from build123d import *

# Parameters (mm, degrees)
ESQUISSE1_R             = 10
BOSS_EXTRU_1_DEPTH      = 1
ESQUISSE2_R             = 6.25
BOSS_EXTRU_2_DEPTH      = 2.5
ESQUISSE3_R             = 3.25
ENL_V_MAT_EXTRU_1_DEPTH = 15.568802284
CHANFREIN1_SIZE         = 0.2


with BuildPart() as part:
    # Esquisse1 → Boss.-Extru.1 (new body)
    with BuildSketch(Plane(origin=(38.31198223, 224.2058109, 0), x_dir=(0.9566700248572155, 0.2911742837884119, 0), z_dir=(0, 0, -1))):
        with Locations(Location((-101.934891402, 203.3355147, 0), (0, 0, 196.92827176))):
            Circle(ESQUISSE1_R)
    extrude(amount=BOSS_EXTRU_1_DEPTH)

    # Esquisse2 → Boss.-Extru.2 (add)
    with BuildSketch(Plane.XY):
        Circle(ESQUISSE2_R)
    extrude(amount=BOSS_EXTRU_2_DEPTH)

    # Esquisse3 → Enlèv. mat.-Extru.1 (cut, through all)
    with BuildSketch(Plane(origin=(0, 0, -1), x_dir=(1, 0, 0), z_dir=(0, 0, -1))):
        with Locations(Location((0, 0, 0), (0, 0, 270))):
            Circle(ESQUISSE3_R)
    extrude(amount=-ENL_V_MAT_EXTRU_1_DEPTH, mode=Mode.SUBTRACT)

    # Chanfrein1
    chanfrein1_edges = [part.edges().sort_by_distance(p)[0] for p in [
        (-6.25, 0, 2.5),
    ]]
    chamfer(chanfrein1_edges, length=CHANFREIN1_SIZE)


solid = part.part
Work out the finished part from the listing and answer in its coordinate system (mm). Coordinates: 2 decimals unless noted, no trailing zeros. Write each loop counter-clockwise with the first axis right and the second up, starting at its lowest first coordinate (ties: lowest second). Pieces come first, ordered by that corner, then holes.
1. The part is cut by section C-C, the plane z = -0.4. Write down the section's boundary in (x, y), and give its area (3 significant figures).
Results list:
outline: circle Ø20 at (0, 0); hole circle Ø6.5 at (0, 0)
area: 281 mm2
2. For a pull along X with two mould halves and no side action, classify faces 1 (the flat face through (5, -4, 0)), 2 (the cylindrical face through (-1.978, -2.579, 0.726)), 3 (the cylindrical face through (5.96, 1.88, 1.13)) as +X half, -X half, draft (parallel to the pull), parting line (faces both ways), or undercut.
Results list:
face 1: draft
face 2: undercut
face 3: parting line
3. The part is cut by section D-D, the plane z = 1.6. Write down the section's boundary in (x, y).
Results list:
outline: circle Ø12.5 at (0, 0); hole circle Ø6.5 at (0, 0)
4. Consider line 1 along Z through (x, y) = (-3, 7); line 2 along X through (y, z) = (1.75, 0.1); line 3 along Y through (x, z) = (0.5, 1.9). Determine where each line is inside the solid, lowest interval first.
Results list:
line 1: z = -1 to 0
line 2: x = -6 to -2.74, 2.74 to 6
line 3: y = -6.23 to -3.21, 3.21 to 6.23
5. A flat-ended cylindrical pin translates along its axis: pin 1 (1 mm diameter, centred on x = 8, z = 0, fed in from +Y). Find the tip coordinate at first contact, or state that the pin passes through.
Results list:
pin 1: stops at y = 6.61
6. The part is cut by section A-A, the plane x = 0. Write down the section's boundary in (y, z), and give its area (3 significant figures).
Results list:
outline: (-10, -1) - (-3.25, -1) - (-3.25, 2.5) - (-6.05, 2.5) - (-6.25, 2.3) - (-6.25, 0) - (-10, 0) - close; (3.25, -1) - (10, -1) - (10, 0) - (6.25, 0) - (6.25, 2.3) - (6.05, 2.5) - (3.25, 2.5) - close
area: 28.5 mm2
